Here's how the part is built. I have some questions about the finished solid (model axes, mm). A direction names the side the tool comes from. Give positions to 0.01 mm unless a question says otherwise; leave off trailing zeros. Loops run counter-clockwise (first coordinate to the right, second up) from the corner with the lowest first, then second, coordinate; pieces in that order, holes last. Notation, with made-up numbers: (34.25, -18) -> (80.25, -18) arc R15 cw to (80.25, 9) -> close; hole circle Ø5 at (52, 34). An arc over 180 degrees is marked (long way). Answer in a Markdown table with one row per item. Add a question column.
Item 1: If we section it at A-A (z = -28.5): Write out the boundary of the cut face in (x, y).
Item 2: If we section it at D-D (x = -3): Write out the boundary of the cut face in (y, z).
Item 3: We'd pull the mould along Z, two halves only. Please class faces 4 (the face through (3, 4, -19)), 5 (the face through (-1.65, 2, -23)), 6 (the face through (-0.15, 1.97, 6.65)), 7 (the face through (-4.43, 1.97, -37.9)): released by +Z, released by -Z, zero draft, split by the parting line, or undercut.
Item 4: If I drill on line 1 (Z direction, x = 0, y = 0.55); line 2 (Z direction, x = 0, y = 2.7); line 3 (X direction, y = 3, z = 0), over which ranges is the centre line in solid material (lowest first)?
Item 5: Which directions (+Z, -Z, +X, -X, +Y, -Y) give clear straight access to the entire face, cutting with the end or side of a thin tool? Please do faces 1 (the face through (-0.878, 2.378, 3.954)), 2 (the face through (-0.04, 1.97, -40.65)), 3 (the face through (6.65, 2, -18)).
Item 6: For P1, Ø2.5, axis at x = 1, z = -1.5, coming from the +Y side, with a flat end and sliding along its axis, tell me the tip position at first contact or that it passes through.
Item 7: If we section it at C-C (x = 1): Write out the boundary of the cut face in (y, z).
Item 8: If we section it at B-B (y = 2.75): Write out the boundary of the cut face in (x, z), then the cut area to 3 significant figures.
```python
from build123d import *

# Parameters (mm, degrees)
SKETCH1_R           = 6.65
SKETCH1_R_2         = 4.05
BOSS_EXTRUDE1_DEPTH = 4
SKETCH2_R           = 4.05
BOSS_EXTRUDE2_DEPTH = 0.8
SKETCH3_R           = 3.5
CUT_EXTRUDE1_DEPTH  = 1.8
CUT_EXTRUDE2_DEPTH  = 5


with BuildPart() as part:
    # Sketch1 → Boss-Extrude1 (new body)
    with BuildSketch(Plane(origin=(0, 0, 0), x_dir=(1, 0, 0), z_dir=(0, 1, 0))):
        with BuildLine():
            Line((-6.65, 36.5), (-6.65, 0))
            ThreePointArc((-6.65, 0), (-4.702260096, 4.702260094), (-2e-09, 6.65))
            ThreePointArc((-2e-09, 6.65), (4.702260094, 4.702260096), (6.65, 0))
            Line((6.65, 0), (6.65, 36.5))
            ThreePointArc((6.65, 36.5), (0, 43.15), (-6.65, 36.5))
        make_face()
        with BuildLine():
            ThreePointArc((1.65, 8.3), (1.166726188, 7.13327381), (-2e-09, 6.65))
            ThreePointArc((-2e-09, 6.65), (-1.16672619, 7.133273812), (-1.65, 8.3))
            Line((-1.65, 8.3), (-1.65, 39))
            ThreePointArc((-1.65, 39), (0, 40.65), (1.65, 39))
            Line((1.65, 39), (1.65, 8.3))
        make_face(mode=Mode.SUBTRACT)
        Circle(SKETCH1_R)
        Circle(SKETCH1_R_2, mode=Mode.SUBTRACT)
    extrude(amount=BOSS_EXTRUDE1_DEPTH)

    # Sketch2 → Boss-Extrude2 (add)
    with BuildSketch(Plane(origin=(0, 0, 0), x_dir=(1, 0, 0), z_dir=(0, 1, 0))):
        Circle(SKETCH2_R)
    extrude(amount=BOSS_EXTRUDE2_DEPTH)

    # Sketch3 → Cut-Extrude1 (cut, through all)
    with BuildSketch(Plane(origin=(0, 0.8, 0), x_dir=(1, 0, 0), z_dir=(0, 1, 0))):
        Circle(SKETCH3_R)
    extrude(amount=-CUT_EXTRUDE1_DEPTH, mode=Mode.SUBTRACT)

    # Sketch4 → Cut-Extrude2 (cut, through all)
    with BuildSketch(Plane.XZ):
        with BuildLine():
            Line((-6.65, -33.142571947), (-2.15, -42.792853089))
            ThreePointArc((-2.15, -42.792853089), (-5.409251335, -40.368139087), (-6.65, -36.5))
            Line((-6.65, -36.5), (-6.65, -33.142571947))
        make_face()
    extrude(amount=-CUT_EXTRUDE2_DEPTH, mode=Mode.SUBTRACT)


solid = part.part
```
Recorded:
| question | item | result |
|---|---|---|
| 1 | outline | (-6.65, 0) -> (-1.65, 0) -> (-1.65, 4) -> (-6.65, 4) -> close; (1.65, 0) -> (6.65, 0) -> (6.65, 4) -> (1.65, 4) -> close |
| 2 | outline | (0, -40.97) -> (4, -40.97) -> (4, -2.72) -> (0.8, -2.72) -> (0.8, -1.8) -> (0, -1.8) -> close; (0, 1.8) -> (0.8, 1.8) -> (0.8, 2.72) -> (4, 2.72) -> (4, 5.93) -> (0, 5.93) -> close |
| 3 | face 4 | zero draft |
| 3 | face 5 | undercut |
| 3 | face 6 | released by +Z |
| 3 | face 7 | released by -Z |
| 4 | line 1 | z = -43.15 to -40.65, -6.65 to -3.5, 3.5 to 6.65 |
| 4 | line 2 | z = -43.15 to -40.65, -6.65 to -4.05, 4.05 to 6.65 |
| 4 | line 3 | x = -6.65 to -4.05, 4.05 to 6.65 |
| 5 | face 1 | +Y |
| 5 | face 2 | +Y, -Y |
| 5 | face 3 | +Z, -Z, +X, +Y, -Y |
| 6 | P1 | passes through |
| 7 | outline | (0, -43.07) -> (4, -43.07) -> (4, -40.31) -> (0, -40.31) -> close; (0, -6.99) -> (4, -6.99) -> (4, -3.92) -> (0.8, -3.92) -> (0.8, -3.35) -> (0, -3.35) -> close; (0, 3.35) -> (0.8, 3.35) -> (0.8, 3.92) -> (4, 3.92) -> (4, 6.57) -> (0, 6.57) -> close |
| 8 | outline | (-6.65, -33.14) -> (-2.15, -42.79) arc R6.65 ccw to (6.65, -36.5) -> (6.65, 0) arc R6.65 ccw to (-6.65, 0) -> close; hole circle Ø8.1 at (0, 0); hole (-1.65, -39) arc R1.65 ccw to (1.65, -39) -> (1.65, -8.3) arc R1.65 ccw to (-1.65, -8.3) -> close |
| 8 | area | 449 mm^2 |
